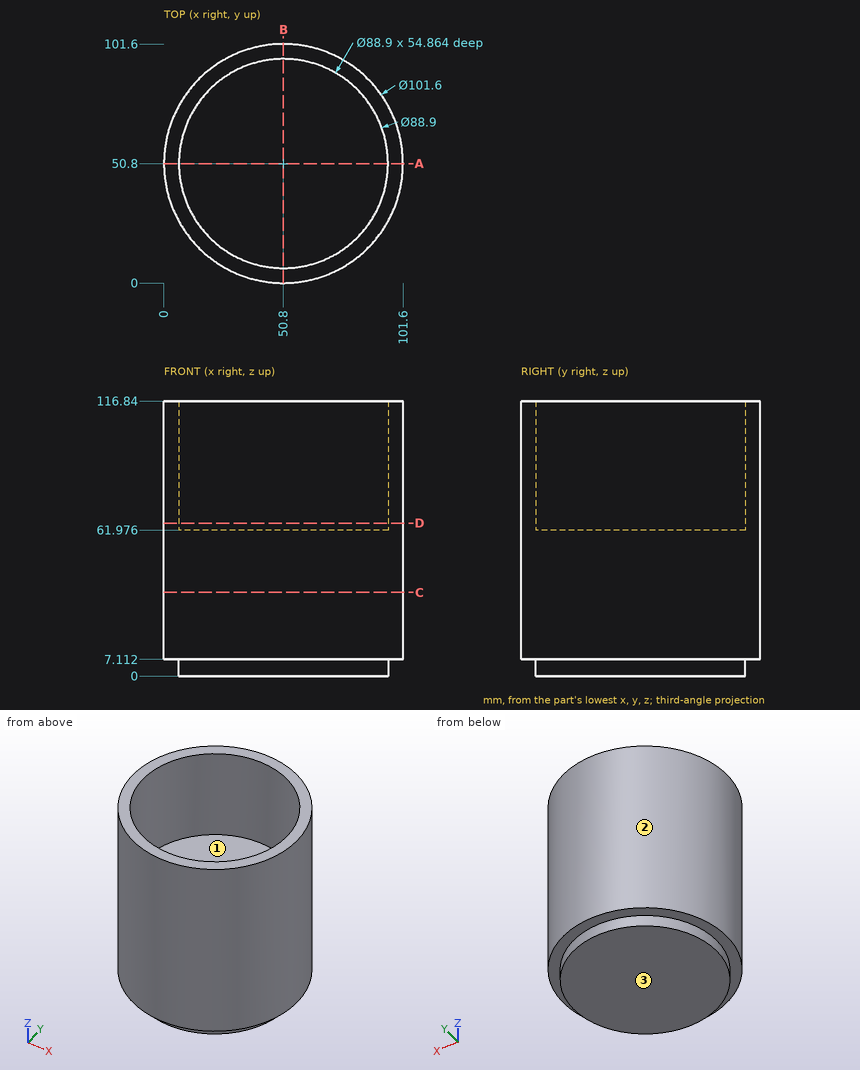
The drawing under review shows one solid part. Ordinate dimensions are in mm from its lowest x, y, z. Coordinates: 2 decimals unless noted, no trailing zeros. Write each loop counter-clockwise with the first axis right and the second up, starting at its lowest first coordinate (ties: lowest second). Pieces come first, ordered by that corner, then holes. Notation, with made-up numbers: (-17.5, -35) - (3.5, -35) arc R17 cw to (3.5, -14) - close; hole circle Ø10 at (74, 47.5). An arc over 180 degrees is marked (long way). Answer in a Markdown table with one row per item. Add a question column.
Q1. We need section C-C, the plane z = 35.5. State the section outline as (x, y) points.
Q2. We need section A-A, the plane y = 50.8. State the section outline as (x, z) points.
Q3. For P1, Ø12, axis at x = 26, z = 97, coming from the -Y side; P2, Ø2, axis at x = 54.5, z = 14, coming from the +Y side; P3, Ø1.5, axis at y = 67.5, z = 70, coming from the -X side, all flat-tipped, find the tip position at first contact; note any pin that passes through.
Q4. We need section D-D, the plane z = 65. State the section outline as (x, y) points.
Q5. For probe 1 along Y at (x, z) = (50, 106); probe 2 along Z at (x, y) = (51.5, 25), list the stretches that pass through material, from the lowest coordinate up.
Q6. Draft analysis for pull direction X (two halves, no side actions). For the marked faces 1, 2 and 3, state which applies: +X half, -X half, draft (parallel to the pull), parting line (faces both ways), or undercut.
Answer list:
| question | item | result |
|---|---|---|
| 1 | outline | circle Ø101.6 at (50.8, 50.8) |
| 2 | outline | (0, 7.11) - (6.35, 7.11) - (6.35, 0) - (95.25, 0) - (95.25, 7.11) - (101.6, 7.11) - (101.6, 116.84) - (95.25, 116.84) - (95.25, 61.98) - (6.35, 61.98) - (6.35, 116.84) - (0, 116.84) - close |
| 3 | P1 | stops at y = 3.61 |
| 3 | P2 | stops at y = 101.53 |
| 3 | P3 | stops at x = 2.57 |
| 4 | outline | circle Ø101.6 at (50.8, 50.8); hole circle Ø88.9 at (50.8, 50.8) |
| 5 | probe 1 | y = 0.01 to 6.36, 95.24 to 101.59 |
| 5 | probe 2 | z = 0 to 61.98 |
| 6 | face 1 | undercut |
| 6 | face 2 | parting line |
| 6 | face 3 | draft |
